Could you check a few things on this model? Use its own coordinates, in mm. Give positions to 0.01 mm unless a question says otherwise; leave off trailing zeros. Write each loop counter-clockwise with the first axis right and the second up, starting at its lowest first coordinate (ties: lowest second). Pieces come first, ordered by that corner, then holes. Notation, with made-up numbers: M 17,-12.5 L 74,-12.5 A5 ccw 74,-6.5 Z; hole C 69,38.25 d6. An arc over 180 degrees is marked long. Use one line per item in the form item = value.
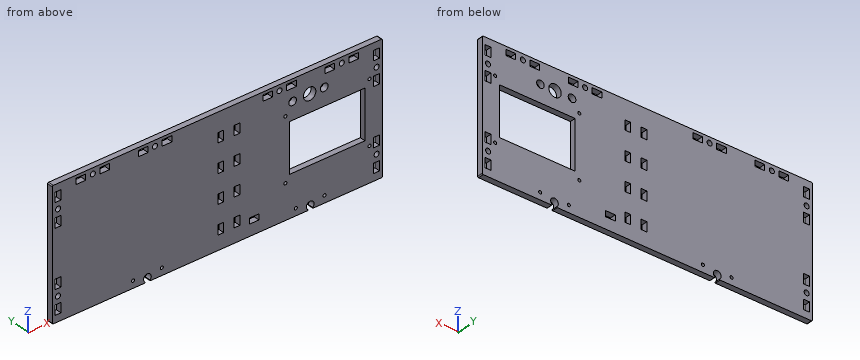
from build123d import *

# Parameters (mm, degrees)
SKETCH1_W                = 344.8
SKETCH1_H                = 134.5
BOSS_EXTRUDE1_DEPTH      = 6
SKETCH2_R                = 6.5
SKETCH2_R_2              = 4
SKETCH2_W                = 78.65
SKETCH2_H                = 51.2
CUT_EXTRUDE1_DEPTH       = 7
M3_CLEARANCE_HOLE1_D     = 3.2
M5_CLEARANCE_HOLE1_D     = 5.3
SKETCH7_W                = 6.1
SKETCH7_H                = 10.1
CUT_EXTRUDE2_DEPTH       = 4
CUT_EXTRUDE2_DEPTH_BACK  = 4
SKETCH71_W               = 6.1
SKETCH71_H               = 10.1
CUT_EXTRUDE21_DEPTH      = 4
CUT_EXTRUDE21_DEPTH_BACK = 4
SKETCH72_W               = 6.1
SKETCH72_H               = 10.1
CUT_EXTRUDE22_DEPTH      = 4
CUT_EXTRUDE22_DEPTH_BACK = 4
SKETCH73_W               = 6.1
SKETCH73_H               = 10.1
CUT_EXTRUDE23_DEPTH      = 4
CUT_EXTRUDE23_DEPTH_BACK = 4
SKETCH74_W               = 6.1
SKETCH74_H               = 10.1
CUT_EXTRUDE24_DEPTH      = 4
CUT_EXTRUDE24_DEPTH_BACK = 4
SKETCH75_W               = 6.1
SKETCH75_H               = 10.1
CUT_EXTRUDE25_DEPTH      = 4
CUT_EXTRUDE25_DEPTH_BACK = 4
SKETCH77_W               = 6.1
SKETCH77_H               = 10.1
CUT_EXTRUDE27_DEPTH      = 4
CUT_EXTRUDE27_DEPTH_BACK = 4
SKETCH78_W               = 6.1
SKETCH78_H               = 10.1
CUT_EXTRUDE28_DEPTH      = 4
CUT_EXTRUDE28_DEPTH_BACK = 4
CUT_EXTRUDE29_DEPTH      = 7
SKETCH62_W               = 10
SKETCH62_H               = 6
CUT_EXTRUDE12_DEPTH      = 4
SKETCH63_W               = 10
SKETCH63_H               = 6
CUT_EXTRUDE13_DEPTH      = 4
SKETCH64_W               = 10
SKETCH64_H               = 6
CUT_EXTRUDE14_DEPTH      = 4
SKETCH65_W               = 10
SKETCH65_H               = 6
CUT_EXTRUDE15_DEPTH      = 4
SKETCH81_R               = 2.65
BOSS_EXTRUDE2_DEPTH      = 6
SKETCH67_W               = 10
SKETCH67_H               = 6
CUT_EXTRUDE17_DEPTH      = 4
CUT_EXTRUDE17_DEPTH_BACK = 4
M3_CLEARANCE_HOLE2_D     = 3.2
FILLET1_R                = 1


with BuildPart() as part:
    # Sketch1 → Boss-Extrude1 (new body)
    with BuildSketch(Plane(origin=(0, 0, 0), x_dir=(1, 0, 0), z_dir=(0, 1, 0))):
        Rectangle(SKETCH1_W, SKETCH1_H)
    extrude(amount=BOSS_EXTRUDE1_DEPTH)

    # Sketch2 → Cut-Extrude1 (cut, through all)
    with BuildSketch(Plane(origin=(0, 0, 0), x_dir=(-1, 0, 0), z_dir=(0, -1, 0))):
        with Locations((-96.4, -45.25)):
            Circle(SKETCH2_R)
        with Locations((-78.65, -45.25)):
            Circle(SKETCH2_R_2)
        with Locations((-111.65, -45.25)):
            Circle(SKETCH2_R_2)
        with Locations((-114.825, -1.4)):
            Rectangle(SKETCH2_W, SKETCH2_H)
    extrude(amount=-CUT_EXTRUDE1_DEPTH, mode=Mode.SUBTRACT)

    # M3 Clearance Hole1 (through all)
    with Locations(Plane(origin=(0, 0, 0), x_dir=(-1, 0, 0), z_dir=(0, -1, 0))):
        with Locations((-159, 31.1), (-71.05, 31.1), (-71.05, -33.9), (-159, -33.9)):
            Hole(M3_CLEARANCE_HOLE1_D / 2)

    # M5 Clearance Hole1 (through all)
    with Locations(Plane(origin=(0, 0, 0), x_dir=(-1, 0, 0), z_dir=(0, -1, 0))):
        with Locations((0, -61.25), (65, -61.25), (130, -61.25), (-166.4, -42.25), (-166.4, 42.25)):
            m5_clearance_hole1 = Hole(M5_CLEARANCE_HOLE1_D / 2)

    # Mirror1: M5 Clearance Hole1 across plane
    add(m5_clearance_hole1.mirror(Plane(origin=(0, 0, 0), x_dir=(0, 0, 1), z_dir=(1, 0, 0))), mode=Mode.SUBTRACT)

    # Sketch7 → Cut-Extrude2 (cut, two sides)
    with BuildSketch(Plane(origin=(122.4, 3, -22.25), x_dir=(1, 0, 0), z_dir=(0, -1, 0))) as cut_extrude2_sk:
        with Locations((44, -32.5)):
            Rectangle(SKETCH7_W, SKETCH7_H)
        with Locations((44, -7.5)):
            Rectangle(SKETCH7_W, SKETCH7_H)
    extrude(amount=CUT_EXTRUDE2_DEPTH, mode=Mode.SUBTRACT)
    extrude(cut_extrude2_sk.sketch, amount=-CUT_EXTRUDE2_DEPTH_BACK, mode=Mode.SUBTRACT)

    # Sketch71 → Cut-Extrude21 (cut, two sides)
    with BuildSketch(Plane(origin=(122.4, 3, 62.25), x_dir=(1, 0, 0), z_dir=(0, -1, 0))) as cut_extrude21_sk:
        with Locations((44, -32.5)):
            Rectangle(SKETCH71_W, SKETCH71_H)
        with Locations((44, -7.5)):
            Rectangle(SKETCH71_W, SKETCH71_H)
    extrude(amount=CUT_EXTRUDE21_DEPTH, mode=Mode.SUBTRACT)
    extrude(cut_extrude21_sk.sketch, amount=-CUT_EXTRUDE21_DEPTH_BACK, mode=Mode.SUBTRACT)

    # Sketch72 → Cut-Extrude22 (cut, two sides)
    with BuildSketch(Plane(origin=(-210.4, 3, -22.25), x_dir=(1, 0, 0), z_dir=(0, -1, 0))) as cut_extrude22_sk:
        with Locations((44, -32.5)):
            Rectangle(SKETCH72_W, SKETCH72_H)
        with Locations((44, -7.5)):
            Rectangle(SKETCH72_W, SKETCH72_H)
    extrude(amount=CUT_EXTRUDE22_DEPTH, mode=Mode.SUBTRACT)
    extrude(cut_extrude22_sk.sketch, amount=-CUT_EXTRUDE22_DEPTH_BACK, mode=Mode.SUBTRACT)

    # Sketch73 → Cut-Extrude23 (cut, two sides)
    with BuildSketch(Plane(origin=(-210.4, 3, 62.25), x_dir=(1, 0, 0), z_dir=(0, -1, 0))) as cut_extrude23_sk:
        with Locations((44, -32.5)):
            Rectangle(SKETCH73_W, SKETCH73_H)
        with Locations((44, -7.5)):
            Rectangle(SKETCH73_W, SKETCH73_H)
    extrude(amount=CUT_EXTRUDE23_DEPTH, mode=Mode.SUBTRACT)
    extrude(cut_extrude23_sk.sketch, amount=-CUT_EXTRUDE23_DEPTH_BACK, mode=Mode.SUBTRACT)

    # Sketch74 → Cut-Extrude24 (cut, two sides)
    with BuildSketch(Plane(origin=(150, 3, 105.25), x_dir=(0, 0, -1), z_dir=(0, -1, 0))) as cut_extrude24_sk:
        with Locations((44, -32.5)):
            Rectangle(SKETCH74_W, SKETCH74_H)
        with Locations((44, -7.5)):
            Rectangle(SKETCH74_W, SKETCH74_H)
    extrude(amount=CUT_EXTRUDE24_DEPTH, mode=Mode.SUBTRACT)
    extrude(cut_extrude24_sk.sketch, amount=-CUT_EXTRUDE24_DEPTH_BACK, mode=Mode.SUBTRACT)

    # Sketch75 → Cut-Extrude25 (cut, two sides)
    with BuildSketch(Plane(origin=(45, 3, 17.25), x_dir=(0, 0, 1), z_dir=(0, -1, 0))) as cut_extrude25_sk:
        with Locations((44, -32.5)):
            Rectangle(SKETCH75_W, SKETCH75_H)
        with Locations((44, -7.5)):
            Rectangle(SKETCH75_W, SKETCH75_H)
    extrude(amount=CUT_EXTRUDE25_DEPTH, mode=Mode.SUBTRACT)
    extrude(cut_extrude25_sk.sketch, amount=-CUT_EXTRUDE25_DEPTH_BACK, mode=Mode.SUBTRACT)

    # Sketch77 → Cut-Extrude27 (cut, two sides)
    with BuildSketch(Plane(origin=(-85, 3, 17.25), x_dir=(0, 0, 1), z_dir=(0, -1, 0))) as cut_extrude27_sk:
        with Locations((44, -32.5)):
            Rectangle(SKETCH77_W, SKETCH77_H)
        with Locations((44, -7.5)):
            Rectangle(SKETCH77_W, SKETCH77_H)
    extrude(amount=CUT_EXTRUDE27_DEPTH, mode=Mode.SUBTRACT)
    extrude(cut_extrude27_sk.sketch, amount=-CUT_EXTRUDE27_DEPTH_BACK, mode=Mode.SUBTRACT)

    # Sketch78 → Cut-Extrude28 (cut, two sides)
    with BuildSketch(Plane(origin=(-150, 3, 17.25), x_dir=(0, 0, 1), z_dir=(0, -1, 0))) as cut_extrude28_sk:
        with Locations((44, -32.5)):
            Rectangle(SKETCH78_W, SKETCH78_H)
        with Locations((44, -7.5)):
            Rectangle(SKETCH78_W, SKETCH78_H)
    extrude(amount=CUT_EXTRUDE28_DEPTH, mode=Mode.SUBTRACT)
    extrude(cut_extrude28_sk.sketch, amount=-CUT_EXTRUDE28_DEPTH_BACK, mode=Mode.SUBTRACT)

    # Sketch79 → Cut-Extrude29 (cut, through all)
    with BuildSketch(Plane(origin=(0, 0, 0), x_dir=(-1, 0, 0), z_dir=(0, -1, 0))):
        with BuildLine():
            Line((-100.023715784, 67.25), (-93.976284216, 67.25))
            ThreePointArc((-93.976284216, 67.25), (-94.5108067, 66.880601937), (-94.354248689, 66.25))
            ThreePointArc((-94.354248689, 66.25), (-97, 59.25), (-99.645751311, 66.25))
            ThreePointArc((-99.645751311, 66.25), (-99.4891933, 66.880601937), (-100.023715784, 67.25))
        make_face()
    cut_extrude29 = extrude(amount=-CUT_EXTRUDE29_DEPTH, mode=Mode.SUBTRACT)

    # Mirror3: Cut-Extrude29 across plane
    add(cut_extrude29.mirror(Plane.ZY.offset(-12)), mode=Mode.SUBTRACT)

    # Sketch62 → Cut-Extrude12 (cut, symmetric)
    with BuildSketch(Plane(origin=(-40.5, 3, 41.482221392), x_dir=(0, 0, 1), z_dir=(0, -1, 0))):
        with Locations((0.767778608, -44)):
            Rectangle(SKETCH62_W, SKETCH62_H)
    cut_extrude12 = extrude(amount=CUT_EXTRUDE12_DEPTH, both=True, mode=Mode.SUBTRACT)

    # Sketch63 → Cut-Extrude13 (cut, symmetric)
    with BuildSketch(Plane(origin=(-40.5, 3, 11.648888059), x_dir=(0, 0, 1), z_dir=(0, -1, 0))):
        with Locations((0.767778608, -44)):
            Rectangle(SKETCH63_W, SKETCH63_H)
    cut_extrude13 = extrude(amount=CUT_EXTRUDE13_DEPTH, both=True, mode=Mode.SUBTRACT)

    # Sketch64 → Cut-Extrude14 (cut, symmetric)
    with BuildSketch(Plane(origin=(-40.5, 3, -18.184445274), x_dir=(0, 0, 1), z_dir=(0, -1, 0))):
        with Locations((0.767778608, -44)):
            Rectangle(SKETCH64_W, SKETCH64_H)
    cut_extrude14 = extrude(amount=CUT_EXTRUDE14_DEPTH, both=True, mode=Mode.SUBTRACT)

    # Sketch65 → Cut-Extrude15 (cut, symmetric)
    with BuildSketch(Plane(origin=(-40.5, 3, -48.017778608), x_dir=(0, 0, 1), z_dir=(0, -1, 0))):
        with Locations((0.767778608, -44)):
            Rectangle(SKETCH65_W, SKETCH65_H)
    cut_extrude15 = extrude(amount=CUT_EXTRUDE15_DEPTH, both=True, mode=Mode.SUBTRACT)

    # Mirror2: Cut-Extrude12, Cut-Extrude13, Cut-Extrude14, Cut-Extrude15 across plane
    add(cut_extrude12.mirror(Plane(origin=(12, 0, 0), x_dir=(0, 0, 1), z_dir=(1, 0, 0))), mode=Mode.SUBTRACT)
    add(cut_extrude13.mirror(Plane(origin=(12, 0, 0), x_dir=(0, 0, 1), z_dir=(1, 0, 0))), mode=Mode.SUBTRACT)
    add(cut_extrude14.mirror(Plane(origin=(12, 0, 0), x_dir=(0, 0, 1), z_dir=(1, 0, 0))), mode=Mode.SUBTRACT)
    add(cut_extrude15.mirror(Plane(origin=(12, 0, 0), x_dir=(0, 0, 1), z_dir=(1, 0, 0))), mode=Mode.SUBTRACT)

    # Sketch81 → Boss-Extrude2 (add, through all)
    with BuildSketch(Plane.XZ):
        with Locations((0, 61.25)):
            Circle(SKETCH81_R)
    extrude(amount=-BOSS_EXTRUDE2_DEPTH)

    # Sketch67 → Cut-Extrude17 (cut, two sides)
    with BuildSketch(Plane(origin=(37.732221392, 3, -8.25), x_dir=(1, 0, 0), z_dir=(0, -1, 0))) as cut_extrude17_sk:
        with Locations((0.767778608, -44)):
            Rectangle(SKETCH67_W, SKETCH67_H)
    extrude(amount=CUT_EXTRUDE17_DEPTH, mode=Mode.SUBTRACT)
    extrude(cut_extrude17_sk.sketch, amount=-CUT_EXTRUDE17_DEPTH_BACK, mode=Mode.SUBTRACT)

    # M3 Clearance Hole2 (through all)
    with Locations(Plane(origin=(0, 0, 0), x_dir=(-1, 0, 0), z_dir=(0, -1, 0))):
        with Locations((-112, 59.75), (-82, 59.75), (58, 59.75), (88, 59.75)):
            Hole(M3_CLEARANCE_HOLE2_D / 2)

    # Fillet1
    fillet1_edges = [part.edges().sort_by_distance(p)[0] for p in [
        (172.4, 3, 67.25),
        (-172.4, 3, 67.25),
        (-172.4, 3, -67.25),
        (172.4, 3, -67.25),
    ]]
    fillet(fillet1_edges, radius=FILLET1_R)


solid = part.part
1) I want a section at C-C, the plane y = 2.35. Count the separate pieces of the cut face and the enclosed holes in it, plus the area to 3 significant figures.
Checked values:
separate_pieces = 1
enclosed_holes = 45
area = 40,200 mm2
2) I want a section at B-B, the plane z = -8. Please give me the cut outline in (x, y).
Checked values:
outline = M -172.4,0 L 75.5,0 L 75.5,6 L -172.4,6 Z; M 154.15,0 L 172.4,0 L 172.4,6 L 154.15,6 Z
3) If I drill on L1, parallel to X at y = 3.55, z = 45.25; L2, parallel to X at y = 0.5, z = 57; L3, parallel to X at y = 3.1, z = -63.25, over which ranges is the centre line in solid material (lowest first)?
Checked values:
L1 = -172.4 to 0.5, 6.5 to 17.5, 23.5 to 74.65, 82.65 to 89.9, 102.9 to 107.65, 115.65 to 172.4
L2 = -172.4 to -169.45, -163.35 to 163.35, 169.45 to 172.4
L3 = -172.4 to -77, -69 to 93, 101 to 172.4
4) I want a section at A-A, the plane x = 38.5. Please give me the cut outline in (y, z).
Checked values:
outline = M 0,-67.25 L 6,-67.25 L 6,-55.25 L 0,-55.25 Z; M 0,-49.25 L 6,-49.25 L 6,67.25 L 0,67.25 Z
5) For pin 1 Ø3 at (x, z) = (166.4, -42.25) entering from -Y, with a flat end and sliding along its axis, tell me the tip position at first contact or that it passes through.
Checked values:
pin_1 = through
